Can you work these out from the model? Positions are in its coordinate system, mm. Give positions to 0.01 mm unless a question says otherwise; leave off trailing zeros. Write each loop counter-clockwise with the first axis right and the second up, starting at its lowest first coordinate (ties: lowest second). Pieces come first, ordered by that corner, then holes.
```python
from build123d import *

# Parameters (mm, degrees)
F0_R     = 2.8575
F1_DEPTH = 76.2
F0_R_2   = 4.445
F2_DEPTH = 1.905
F0_R_3   = 6.35
F3_DEPTH = 3.81


with BuildPart() as f1:
    # F0 (on Top) → F1 (new body)
    with BuildSketch(Plane.XY):
        Circle(F0_R)
    extrude(amount=F1_DEPTH)

    # F0 (on Top) → F2 (join, symmetric)
    with BuildSketch(Plane.XY):
        Circle(F0_R_2)
        Circle(F0_R, mode=Mode.SUBTRACT)
    extrude(amount=F2_DEPTH, both=True)

    # F0 (on Top) → F3 (join)
    with BuildSketch(Plane.XY):
        Circle(F0_R_3)
        Circle(F0_R_2, mode=Mode.SUBTRACT)
    extrude(amount=-F3_DEPTH)


solid = f1.part
```
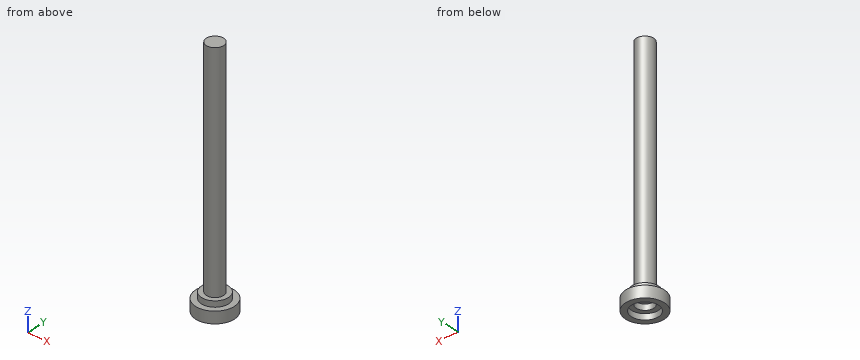
1) For pin 1 Ø4 at (y, z) = (3, 5) entering from -X; pin 2 Ø3 at (x, y) = (0, -0.5) entering from -Z; pin 3 Ø6 at (y, z) = (-0.5, 9) entering from -X, each with a flat end and sliding along its axis, tell me the tip position at first contact or that it passes through.
Values follow:
pin 1: stops at x = -2.68
pin 2: stops at z = 0
pin 3: stops at x = -2.86
2) Please list where these lines run through material, in increasing order: L1, parallel to Y at x = 0, z = -1.05; L2, parallel to Z at x = -1.5, y = 1.25; L3, parallel to Z at x = 5, y = -3.
Values follow:
L1: y = -6.35 to -2.86, 2.86 to 6.35
L2: z = 0 to 76.2
L3: z = -3.81 to 0
3) Suppose I cut it at C-C on z = 3. Write out the boundary of the cut face in (x, y) (1 decimal), plus the area to 3 significant figures.
Values follow:
outline: circle Ø5.7 at (0, 0)
area: 25.7 mm2
